Geometry: see drawing. Coordinates: mm, zero at the bounding-box minimum. A direction names the side the tool comes from. Give positions to 0.01 mm unless a question says otherwise; leave off trailing zeros. Order: outer loops, then holes, each group sorted by start corner. A loop starts at its lowest first (then second) coordinate and runs counter-clockwise, first axis right, second up. Notation, with made-up numbers: M -21,-13 L 3,-13 A17 ccw 3,11 Z; hole C -11.5,-7.5 d3. An arc over 180 degrees is marked long. Use a Markdown table: item, result.
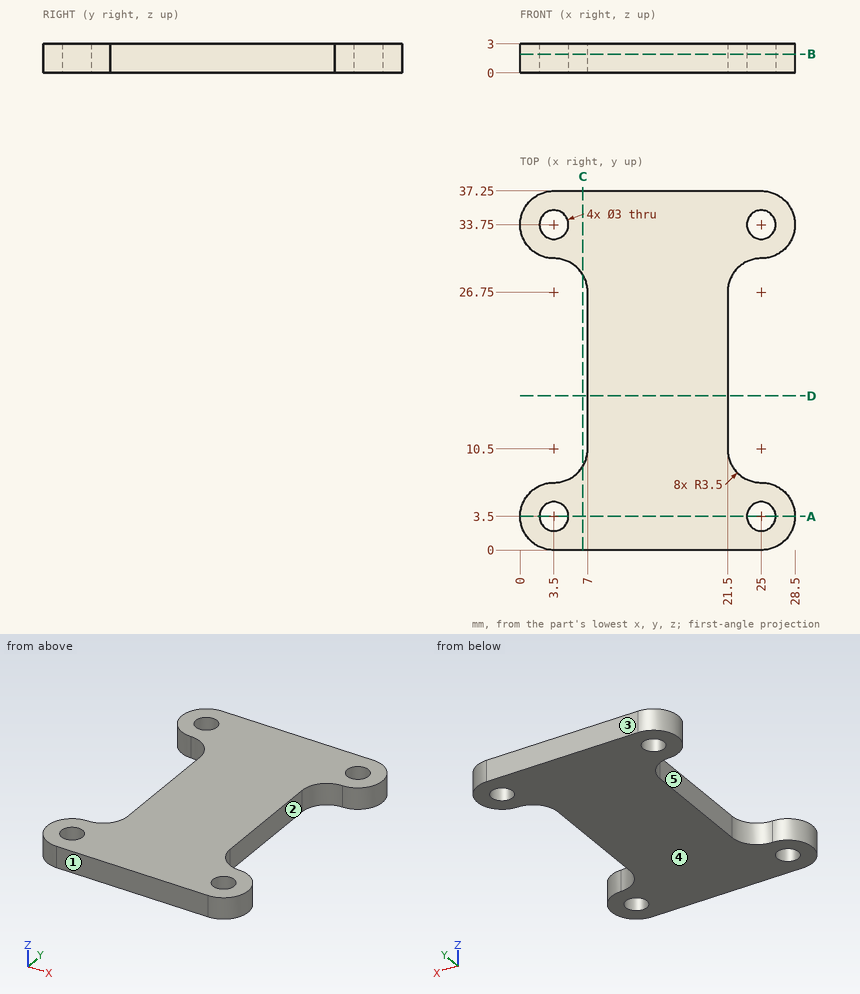
1) First-contact query: pin 1 Ø0.9 at (y, z) = (18.5, 2) entering from -X. Flat tip, straight axial feed; report the tip coordinate or a pass-through.
Response values:
| item | result |
|---|---|
| pin 1 | stops at x = 7 |
2) Reachability of the marked faces 4 and 5 from +Z, -Z, +X, -X, +Y, -Y: full face, straight path, thin tool, end or side. Return the list, or none.
Response values:
| item | result |
|---|---|
| face 4 | -Z, +X, -X, +Y, -Y |
| face 5 | +Z, -Z, -X |
3) Cut plane B-B on z = 1.95. Return loops of the section in (x, y).
Response values:
| item | result |
|---|---|
| outline | M 3.5,0 L 25,0 A3.5 ccw 25,7 A3.5 cw 21.5,10.5 L 21.5,26.75 A3.5 cw 25,30.25 A3.5 ccw 25,37.25 L 3.5,37.25 A3.5 ccw 3.5,30.25 A3.5 cw 7,26.75 L 7,10.5 A3.5 cw 3.5,7 A3.5 ccw Z; hole C 3.5,3.5 d3; hole C 3.5,33.75 d3; hole C 25,3.5 d3; hole C 25,33.75 d3 |
4) Cut plane C-C on x = 6.5. Return loops of the section in (y, z), and give its area (3 significant figures).
Response values:
| item | result |
|---|---|
| outline | M 0,0 L 8.7,0 L 8.7,3 L 0,3 Z; M 28.55,0 L 37.25,0 L 37.25,3 L 28.55,3 Z |
| area | 52.2 mm² |
5) Cut plane A-A on y = 3.5. Return loops of the section in (x, z).
Response values:
| item | result |
|---|---|
| outline | M 0,0 L 2,0 L 2,3 L 0,3 Z; M 5,0 L 23.5,0 L 23.5,3 L 5,3 Z; M 26.5,0 L 28.5,0 L 28.5,3 L 26.5,3 Z |
6) Material intervals for line 1 (Y direction, x = 3.5, z = 1.2); line 2 (X direction, y = 4.5, z = 0.7), sorted ascending. Write a range as from..to.
Response values:
| item | result |
|---|---|
| line 1 | y = 0..2, 5..7, 30.25..32.25, 35.25..37.25 |
| line 2 | x = 0.15..2.38, 4.62..23.88, 26.12..28.35 |
7) Cut plane D-D on y = 16. Return loops of the section in (x, z), and give its area (3 significant figures).
Response values:
| item | result |
|---|---|
| outline | M 7,0 L 21.5,0 L 21.5,3 L 7,3 Z |
| area | 43.5 mm² |
8) Mould query, pull axis Y, two halves, no side actions, for the marked faces 1, 2 and 3. Classes: released by +Y, released by -Y, zero draft, split by the parting line, or undercut.
Response values:
| item | result |
|---|---|
| face 1 | released by -Y |
| face 2 | undercut |
| face 3 | released by +Y |
